Solid Edge part; units mm, degrees
sketch "Sketch1" plane through (0, 0, 0) normal (1, 0, 0) x (0, 1, 0)
  line L0 (-72.39, 0) -> (-72.39, 3.175)
  line L1 (-72.39, 3.175) -> (-63.5, 3.175)
  line L2 (-63.5, 3.175) -> (-63.5, 12.7)
  line L3 (-63.5, 12.7) -> (25.4, 12.7)
  line L4 (25.4, 12.7) -> (25.4, 4.217)
  line L5 (25.4, 4.217) -> (72.39, 4.217)
  line L6 (72.39, 4.217) -> (72.39, 0)
  line L7 (-72.39, 0) -> (72.39, 0)
revolve "RevolvedProtrusion1" add sketch "Sketch1" angle 360 about axis through (0, -60.0075, 0) along (0, 1, 0)
sketch "Sketch2" plane through (0, 0, 0) normal (1, 0, 0) x (0, 1, 0)
  line L0 (-11.43, 313.69) -> (11.43, 313.69)
  line L1 (11.43, 313.69) -> (12.7, 321.31)
  line L2 (10.2235, 321.31) -> (12.7, 321.31)
  line L3 (10.2235, 317.5) -> (10.2235, 321.31)
  line L4 (-10.2235, 317.5) -> (10.2235, 317.5)
  line L5 (-10.2235, 321.31) -> (-10.2235, 317.5)
  line L6 (-12.7, 321.31) -> (-10.2235, 321.31)
  line L7 (-11.43, 313.69) -> (-12.7, 321.31)
  dimension "D1" = 11.43
revolve "RevolvedProtrusion2" add sketch "Sketch2" angle 360 about axis through (0, -60.0075, 0) along (0, 1, 0)
sketch "Sketch3" plane through (0, 0, 0) normal (0, -1, 0) x (1, 0, 0)
  circle A0 centre (0, 0) radius 313.69
extrude "Protrusion1" add sketch "Sketch3" along normal mid plane 5.08
fillet "Round_1" radius 50.8 2 edges at (0, -2.54, -12.7) (0, 2.54, -12.7)
sketch "Sketch4" plane through (0, -2.54, 0) normal (0, -1, 0) x (1, 0, 0)
  arc A0 (-77.8035, 290.3666) -> (-260.3356, 150.3048) centre (0, 0) ccw
  line L0 (-54.9926, 31.75) -> (-260.3356, 150.3048)
  arc A1 (-16.435, 61.3363) -> (-54.9926, 31.75) centre (0, 0) ccw
  line L1 (-16.435, 61.3363) -> (-77.8035, 290.3666)
extrude "Cutout1" cut sketch "Sketch4" against normal through all
pattern_circular "Pattern1" count 6 over 360 about axis through (0, -2.54, 0) along (0, -1, 0) of "Cutout1"
sketch "Sketch5" plane through (0, 0, 0) normal (0, -1, 0) x (1, 0, 0)
  line L0 (0, 12.7) -> (-12.7, 0)
  line L1 (-12.7, 0) -> (0, -12.7)
  line L2 (0, -12.7) -> (12.7, 0)
  line L3 (12.7, 0) -> (0, 12.7)
extrude "ExtrudedProtrusion_2" add sketch "Sketch5" against normal blind 63.5
properties part number "8-7" material "Carbon Fiber"
The listing builds one solid part. Answer for the finished solid, in the listing's coordinates (mm). A direction names the side the tool comes from. Give positions to 0.01 mm unless a question says otherwise; leave off trailing zeros. Loops run counter-clockwise (first coordinate to the right, second up) from the corner with the lowest first, then second, coordinate; pieces in that order, holes last. Notation, with made-up numbers: (-31, -7.75) - (28, -7.75) arc R18 cw to (28, 4.25) - close; hole circle Ø7 at (88.25, 13). An arc over 180 degrees is marked (long way). Return JSON: item names as keys, results as strings. Group by question number.
1. Find section A-A (z = -112). State how many separate pieces and enclosed holes the cut face has, then the cut area to 3 significant figures.
2. Which of the six approach directions +Z, -Z, +X, -X, +Y, -Y give full straight-line access (tool end or side, diameter ignored) to faces 4 (the flat face through (128, 0, 128)), 5 (the flat face through (-3, -63.5, 3)), 6 (the flat face through (-68, 2.54, 25))?
3. Find section B-B (y = 33). Write down the section's boundary in (x, z).
4. Straight lines are drawn through the part: line 1 (X direction, y = 7.5, z = 0); line 2 (Y direction, x = 40.5, z = 38); line 3 (Y direction, x = -263.5, z = 145.5). For each, find the intervals that lie inside material, in ascending order. Write a range as [from, to].
5. Determine the mould class of faces 1 (the flat face through (73, -10.224, -311)), 2 (the flat face through (46.69, -0.04, -174.25)), 3 (the cylindrical face through (-195.51, 11.48, -254.98)) for opening direction Z: pulls with the +Z half, pulls with the -Z half, needs draft (parallel to the pull), parting line crosses it, or undercut.
6. Given pin 1 Ø4 at (x, z) = (-9, 7.5) entering from +Y; pin 2 Ø14 at (x, z) = (7.5, 8.5) entering from +Y; pin 3 Ø2.5 at (y, z) = (0.5, 238.5) entering from +X; pin 4 Ø7.5 at (x, z) = (1, -5) entering from -Y, each flat-ended and moving along its own axis, determine where each tip first touches the part or whether it passes through.
Verdict:
{
 "1": {"separate pieces": "4", "enclosed holes": "0", "area": "1,370 mm^2"},
 "2": {"face 4": "+Y, -Y", "face 5": "-Y", "face 6": "+Y"},
 "3": {"outline": "(-12.7, 0) - (0, -12.7) - (12.7, 0) - (0, 12.7) - close"},
 "4": {"line 1": "x = [-317.5, -313.69], [-33.23, 33.23], [313.69, 317.5]", "line 2": "y = [-3.17, 2.54]", "line 3": "y = [-2.54, 2.54]"},
 "5": {"face 1": "needs draft", "face 2": "undercut", "face 3": "parting line crosses it"},
 "6": {"pin 1": "stops at y = 25.4", "pin 2": "stops at y = 63.5", "pin 3": "stops at x = 210.99", "pin 4": "stops at y = -72.39"}
}
